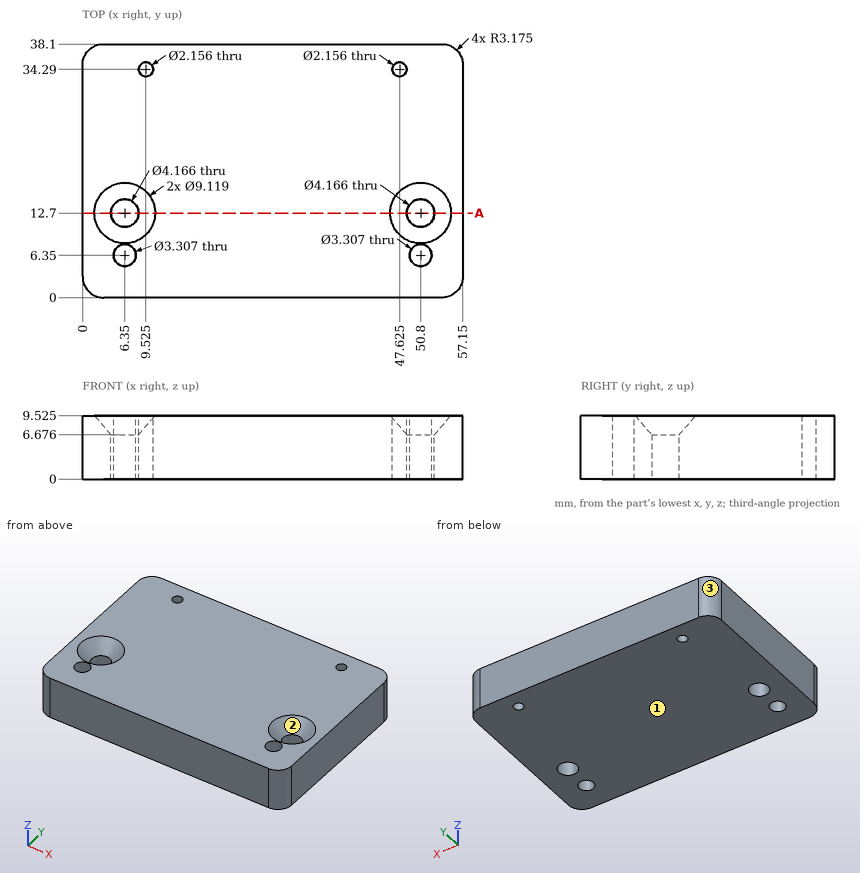
Could you check a few things on this drawing? It's one solid part, dimensions in mm from its lowest x, y, z. Round coordinates to 2 decimals unless told otherwise and drop trailing zeros.
Q1. For P1, Ø5.5, axis at x = 6.35, y = 12.7, coming from the +Z side (1 decimal); P2, Ø1.3, axis at x = 9.525, y = 34.29, coming from the +Z side, each with a flat end and sliding along its axis, tell me the tip position at first contact or that it passes through.
Q2. I want a section at A-A (y = 12.7). Give the number of separate pieces and of enclosed holes in the cut face, and give its area (3 significant figures).
Q3. Please list where these lines run through material, in increasing order: L1, parallel to Y at x = 6.35, z = 4.25; L2, parallel to X at y = 12.7, z = 4.5; L3, parallel to X at y = 34.29, z = 4.75.
Q4. Thinking about a two-plate mould opening in X: for the marked faces 1, 2 and 3, which applies, pulls with the +X half, pulls with the -X half, needs draft (parallel to the pull), parting line crosses it, or undercut?
Answer below:
1. P1: stops at z = 7.4
1. P2: passes through
2. separate pieces: 3
2. enclosed holes: 0
2. area: 451 mm2
3. L1: y = 0 to 4.7, 8 to 10.62, 14.78 to 38.1
3. L2: x = 0 to 4.27, 8.43 to 48.72, 52.88 to 57.15
3. L3: x = 0 to 8.45, 10.6 to 46.55, 48.7 to 57.15
4. face 1: needs draft
4. face 2: undercut
4. face 3: pulls with the -X half
